Geometry check sheet. Reference: drawing and pictorial views, mm from the part's lowest x, y, z. Give positions to 0.01 mm unless a question says otherwise; leave off trailing zeros. Write each loop counter-clockwise with the first axis right and the second up, starting at its lowest first coordinate (ties: lowest second). Pieces come first, ordered by that corner, then holes. Notation, with made-up numbers: (70, -19) -> (78, -19) arc R13 cw to (78, 1) -> close; hole circle Ø2 at (73.5, 4). An arc over 180 degrees is marked (long way). Use a Markdown table: item, result. Add a question column.
1. Cross-section at A-A (x = 32). Enter the section's corners in (y, z), then the cut area to 3 significant figures.
2. Scan lines: probe 1 along Y at (x, z) = (27, 3.6) (3 decimals); probe 2 along Z at (x, y) = (27, 2.6); probe 3 along Y at (x, z) = (15.5, 0.75). Record each from-to range of solid material in increasing order. Write a range as [from, to].
3. Gauge pin test, flat ends, axial feed: P1, Ø1.5, axis at x = 24, z = 3.5, coming from the -Y side; P2, Ø3, axis at x = 31.5, z = 1.5, coming from the +Y side. Record the tip position at first contact, or that the pin passes through.
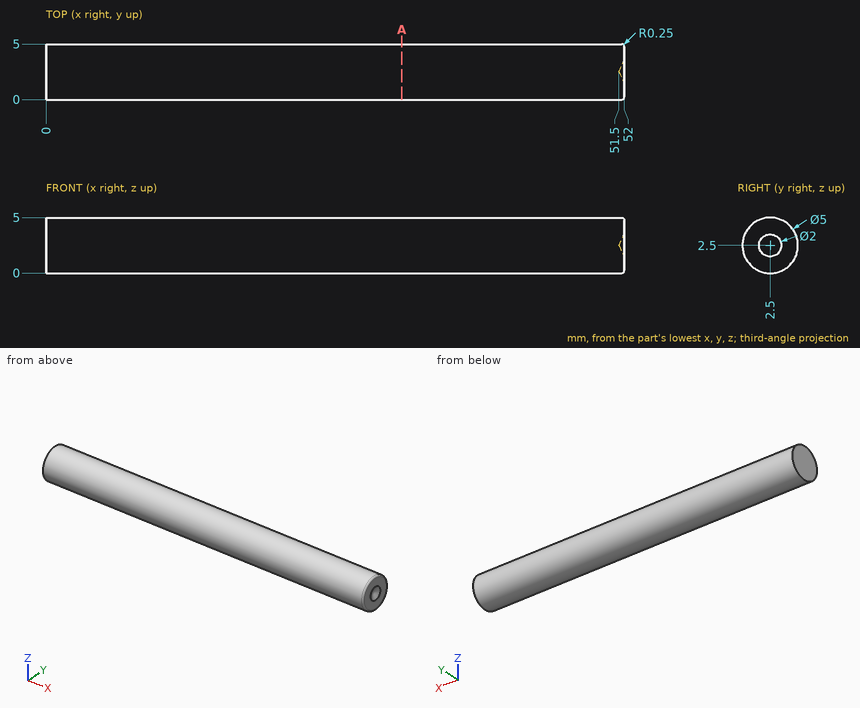
Worked answers:
| question | item | result |
|---|---|---|
| 1 | outline | circle Ø5 at (2.5, 2.5) |
| 1 | area | 19.6 mm² |
| 2 | probe 1 | y = [0.255, 4.745] |
| 2 | probe 2 | z = [0, 5] |
| 2 | probe 3 | y = [0.71, 4.29] |
| 3 | P1 | stops at y = 0.01 |
| 3 | P2 | stops at y = 5 |
